from build123d import *
from build123d.topology import SkipClean

# Parameters (mm, degrees)
BOSS_EXTRUDE1_DEPTH = 25
FILLET1_R           = 2
SKETCH2_R           = 17.5
BOSS_EXTRUDE2_DEPTH = 8
SKETCH3_R           = 16.5
BOSS_EXTRUDE3_DEPTH = 12
SKETCH4_R           = 14.5
CUT_EXTRUDE1_DEPTH  = 2
SKETCH5_R           = 16.5
BOSS_EXTRUDE4_DEPTH = 1
SKETCH6_R           = 2.5
CUT_EXTRUDE2_DEPTH  = 0.75
CUT_EXTRUDE3_DEPTH  = 0.5
CUT_EXTRUDE4_DEPTH  = 0.25
SKETCH11_R          = 5
BOSS_EXTRUDE5_DEPTH = 2
BOSS_EXTRUDE6_DEPTH = 1


with BuildPart() as part:
    # Sketch1 → Boss-Extrude1 (new body)
    with BuildSketch(Plane.XY):
        with BuildLine():
            Line((-32, -20), (32, -20))
            ThreePointArc((32, -20), (34.121320344, -19.121320344), (35, -17))
            Line((35, -17), (35, 17))
            ThreePointArc((35, 17), (34.121320344, 19.121320344), (32, 20))
            Line((32, 20), (-32, 20))
            ThreePointArc((-32, 20), (-34.121320344, 19.121320344), (-35, 17))
            Line((-35, 17), (-35, -17))
            ThreePointArc((-35, -17), (-34.121320344, -19.121320344), (-32, -20))
        make_face()
    extrude(amount=BOSS_EXTRUDE1_DEPTH)

    # Fillet1
    fillet1_edges = [part.edges().sort_by_distance(p)[0] for p in [
        (0, -20, 0),
        (-34.121320344, -19.121320344, 0),
        (-35, 0, 0),
        (-34.121320344, 19.121320344, 0),
        (-34.121320344, -19.121320344, 25),
        (0, -20, 25),
        (34.121320344, -19.121320344, 25),
        (35, 0, 25),
        (34.121320344, 19.121320344, 25),
        (0, 20, 25),
        (-34.121320344, 19.121320344, 25),
        (0, 20, 0),
        (-35, 0, 25),
        (34.121320344, 19.121320344, 0),
        (35, 0, 0),
        (34.121320344, -19.121320344, 0),
    ]]
    fillet(fillet1_edges, radius=FILLET1_R)

    # Sketch2 → Boss-Extrude2 (add)
    with BuildSketch(Plane.XY.offset(25)):
        with Locations(Location((0, 0, 0), (0, 0, 180))):
            Circle(SKETCH2_R)
    extrude(amount=BOSS_EXTRUDE2_DEPTH)

    # Sketch3 → Boss-Extrude3 (add)
    with BuildSketch(Plane.XY.offset(33)):
        Circle(SKETCH3_R)
    extrude(amount=BOSS_EXTRUDE3_DEPTH)

    # Sketch4 → Cut-Extrude1 (cut)
    with BuildSketch(Plane.XY.offset(45)):
        Circle(SKETCH4_R)
    extrude(amount=-CUT_EXTRUDE1_DEPTH, mode=Mode.SUBTRACT)

    # Sketch5 → Boss-Extrude4 (add)
    with BuildSketch(Plane.XY.offset(43)):
        Circle(SKETCH5_R)
    extrude(amount=BOSS_EXTRUDE4_DEPTH)

    # Sketch6 → Cut-Extrude2 (cut)
    with BuildSketch(Plane(origin=(0, 0, 0), x_dir=(-1, 0, 0), z_dir=(0, 0, -1))):
        with Locations((-25, 13.28125)):
            Circle(SKETCH6_R)
        with Locations(Location((25, 13.28125, 0), (0, 0, 180))):
            Circle(SKETCH6_R)
        with Locations((25, -13.28125)):
            Circle(SKETCH6_R)
        with Locations(Location((-25, -13.28125, 0), (0, 0, 180))):
            Circle(SKETCH6_R)
    extrude(amount=-CUT_EXTRUDE2_DEPTH, mode=Mode.SUBTRACT)

    # Sketch7 → Cut-Extrude3 (cut)
    with SkipClean():  # the faces are left unmerged after this step: merging them gives an invalid solid
        with BuildSketch(Plane(origin=(0, 0, 0.75), x_dir=(-1, 0, 0), z_dir=(0, 0, -1))):
            with BuildLine():
                Line((-24.6, 15.749042536), (-24.6, 13.68125))
                Line((-24.6, 13.68125), (-22.532207464, 13.68125))
                ThreePointArc((-22.532207464, 13.68125), (-22.5, 13.28125), (-22.532207464, 12.88125))
                Line((-22.532207464, 12.88125), (-24.6, 12.88125))
                Line((-24.6, 12.88125), (-24.6, 10.813457464))
                ThreePointArc((-24.6, 10.813457464), (-25, 10.78125), (-25.4, 10.813457464))
                Line((-25.4, 10.813457464), (-25.4, 12.88125))
                Line((-25.4, 12.88125), (-27.467792536, 12.88125))
                ThreePointArc((-27.467792536, 12.88125), (-27.5, 13.28125), (-27.467792536, 13.68125))
                Line((-27.467792536, 13.68125), (-25.4, 13.68125))
                Line((-25.4, 13.68125), (-25.4, 15.749042536))
                ThreePointArc((-25.4, 15.749042536), (-25, 15.78125), (-24.6, 15.749042536))
            make_face()
            with BuildLine():
                Line((25.4, 13.68125), (25.4, 15.749042536))
                ThreePointArc((25.4, 15.749042536), (25, 15.78125), (24.6, 15.749042536))
                Line((24.6, 15.749042536), (24.6, 13.68125))
                Line((24.6, 13.68125), (22.532207464, 13.68125))
                ThreePointArc((22.532207464, 13.68125), (22.5, 13.28125), (22.532207464, 12.88125))
                Line((22.532207464, 12.88125), (24.6, 12.88125))
                Line((24.6, 12.88125), (24.6, 10.813457464))
                ThreePointArc((24.6, 10.813457464), (25, 10.78125), (25.4, 10.813457464))
                Line((25.4, 10.813457464), (25.4, 12.88125))
                Line((25.4, 12.88125), (27.467792536, 12.88125))
                ThreePointArc((27.467792536, 12.88125), (27.5, 13.28125), (27.467792536, 13.68125))
                Line((27.467792536, 13.68125), (25.4, 13.68125))
            make_face()
            with BuildLine():
                Line((24.6, -15.749042536), (24.6, -13.68125))
                Line((24.6, -13.68125), (22.532207464, -13.68125))
                ThreePointArc((22.532207464, -13.68125), (22.5, -13.28125), (22.532207464, -12.88125))
                Line((22.532207464, -12.88125), (24.6, -12.88125))
                Line((24.6, -12.88125), (24.6, -10.813457464))
                ThreePointArc((24.6, -10.813457464), (25, -10.78125), (25.4, -10.813457464))
                Line((25.4, -10.813457464), (25.4, -12.88125))
                Line((25.4, -12.88125), (27.467792536, -12.88125))
                ThreePointArc((27.467792536, -12.88125), (27.5, -13.28125), (27.467792536, -13.68125))
                Line((27.467792536, -13.68125), (25.4, -13.68125))
                Line((25.4, -13.68125), (25.4, -15.749042536))
                ThreePointArc((25.4, -15.749042536), (25, -15.78125), (24.6, -15.749042536))
            make_face()
            with BuildLine():
                Line((-25.4, -13.68125), (-25.4, -15.749042536))
                ThreePointArc((-25.4, -15.749042536), (-25, -15.78125), (-24.6, -15.749042536))
                Line((-24.6, -15.749042536), (-24.6, -13.68125))
                Line((-24.6, -13.68125), (-22.532207464, -13.68125))
                ThreePointArc((-22.532207464, -13.68125), (-22.5, -13.28125), (-22.532207464, -12.88125))
                Line((-22.532207464, -12.88125), (-24.6, -12.88125))
                Line((-24.6, -12.88125), (-24.6, -10.813457464))
                ThreePointArc((-24.6, -10.813457464), (-25, -10.78125), (-25.4, -10.813457464))
                Line((-25.4, -10.813457464), (-25.4, -12.88125))
                Line((-25.4, -12.88125), (-27.467792536, -12.88125))
                ThreePointArc((-27.467792536, -12.88125), (-27.5, -13.28125), (-27.467792536, -13.68125))
                Line((-27.467792536, -13.68125), (-25.4, -13.68125))
            make_face()
        extrude(amount=-CUT_EXTRUDE3_DEPTH, mode=Mode.SUBTRACT)

    # Sketch8 → Cut-Extrude4 (cut)
    with SkipClean():  # the faces are left unmerged after this step: merging them gives an invalid solid
        with BuildSketch(Plane(origin=(0, 20, 0), x_dir=(1, 0, 0), z_dir=(0, 1, 0))):
            with BuildLine():
                Line((26, -18), (13, -18))
                ThreePointArc((13, -18), (12.292893219, -17.707106781), (12, -17))
                Line((12, -17), (12, -11))
                ThreePointArc((12, -11), (12.292893219, -10.292893219), (13, -10))
                Line((13, -10), (26, -10))
                ThreePointArc((26, -10), (26.707106781, -10.292893219), (27, -11))
                Line((27, -11), (27, -17))
                ThreePointArc((27, -17), (26.707106781, -17.707106781), (26, -18))
            make_face()
        extrude(amount=-CUT_EXTRUDE4_DEPTH, mode=Mode.SUBTRACT)

    # Sketch11 → Boss-Extrude5 (add)
    with SkipClean():  # the faces are left unmerged after this step: merging them gives an invalid solid
        with BuildSketch(Plane.ZY.offset(35)):
            with Locations(Location((12.5, 0, 0), (0, 0, 180))):
                Circle(SKETCH11_R)
        boss_extrude5 = extrude(amount=BOSS_EXTRUDE5_DEPTH)

    # Mirror1: Boss-Extrude5 across plane
    with SkipClean():  # the faces are left unmerged after this step: merging them gives an invalid solid
        add(boss_extrude5.mirror(Plane(origin=(0, 0, 0), x_dir=(0, 0, 1), z_dir=(1, 0, 0))))

    # Sketch12 → Boss-Extrude6 (add)
    with SkipClean():  # the faces are left unmerged after this step: merging them gives an invalid solid
        with BuildSketch(Plane.XY.offset(25)):
            with BuildLine():
                Line((25.5, 14), (29.5, 14))
                ThreePointArc((29.5, 14), (29.853553391, 13.853553391), (30, 13.5))
                Line((30, 13.5), (30, 12))
                ThreePointArc((30, 12), (29.853553391, 11.646446609), (29.5, 11.5))
                Line((29.5, 11.5), (25.5, 11.5))
                ThreePointArc((25.5, 11.5), (25.146446609, 11.646446609), (25, 12))
                Line((25, 12), (25, 13.5))
                ThreePointArc((25, 13.5), (25.146446609, 13.853553391), (25.5, 14))
            make_face()
        extrude(amount=BOSS_EXTRUDE6_DEPTH)


solid = part.part
Work out the finished part from the listing and answer in its coordinate system (mm). A direction names the side the tool comes from. Give positions to 0.01 mm unless a question says otherwise; leave off trailing zeros. Loops run counter-clockwise (first coordinate to the right, second up) from the corner with the lowest first, then second, coordinate; pieces in that order, holes last. Notation, with made-up numbers: (19, 43.5) - (59, 43.5) arc R22 cw to (59, 64.5) - close; hole circle Ø3 at (-28, 81). An arc over 180 degrees is marked (long way). Answer in a Markdown table with one row per item.
(1) Section A-A (z = 12.5) is taken. Give the vertices of the cut face in (x, y).
Results list:
| item | result |
|---|---|
| outline | (-37, -5) - (-35, -5) - (-35, -17) arc R3 ccw to (-32, -20) - (32, -20) arc R3 ccw to (35, -17) - (35, -5) - (37, -5) - (37, 5) - (35, 5) - (35, 17) arc R3 ccw to (32, 20) - (27, 20) - (27, 19.75) - (12, 19.75) - (12, 20) - (-32, 20) arc R3 ccw to (-35, 17) - (-35, 5) - (-37, 5) - close |
(2) A tool of negligible diameter and unlimited length cuts with its end or side. For faces 5 (the face through (5, -16, 33)), 6 (the face through (-26, 12, 0.75)), 7 (the face through (35.99, -1.5, 7.73)), from which of +Z, -Z, +X, -X, +Y, -Y can it reach the whole face along a straight path? Write none if from no direction.
Results list:
| item | result |
|---|---|
| face 5 | +Z |
| face 6 | -Z |
| face 7 | +X |
(3) For a pull along X with two mould halves and no side action, classify faces 1 (the face through (-34.43, -0.24, 0.6)), 2 (the face through (-26, -14, 0.75)), 3 (the face through (0, 20, 12)), 4 (the face through (26, -12, 0.75)) as pulls with the +X half, pulls with the -X half, needs draft (parallel to the pull), parting line crosses it, or undercut.
Results list:
| item | result |
|---|---|
| face 1 | pulls with the -X half |
| face 2 | undercut |
| face 3 | needs draft |
| face 4 | undercut |
(4) Section C-C (x = 21) is taken. Give the vertices of the cut face in (y, z).
Results list:
| item | result |
|---|---|
| outline | (-20, 2) arc R2 ccw to (-18, 0) - (18, 0) arc R2 ccw to (20, 2) - (20, 10) - (19.75, 10) - (19.75, 18) - (20, 18) - (20, 23) arc R2 ccw to (18, 25) - (-18, 25) arc R2 ccw to (-20, 23) - close |
(5) Section D-D (y = -9) is taken. Give the vertices of the cut face in (x, z).
Results list:
| item | result |
|---|---|
| outline | (-35, 2) arc R2 ccw to (-33, 0) - (33, 0) arc R2 ccw to (35, 2) - (35, 23) arc R2 ccw to (33, 25) - (15.01, 25) - (15.01, 33) - (13.83, 33) - (13.83, 45) - (11.37, 45) - (11.37, 44) - (-11.37, 44) - (-11.37, 45) - (-13.83, 45) - (-13.83, 33) - (-15.01, 33) - (-15.01, 25) - (-33, 25) arc R2 ccw to (-35, 23) - close |
(6) Consider L1, parallel to Y at x = 25, z = 0.2; L2, parallel to Y at x = 0, z = 44.5; L3, parallel to X at y = 15, z = 23. Determine where each line is inside the solid, lowest interval first. Write a range as [from, to].
Results list:
| item | result |
|---|---|
| L1 | y = [-18.87, -15.78], [-10.78, 10.78], [15.78, 18.87] |
| L2 | y = [-16.5, -14.5], [14.5, 16.5] |
| L3 | x = [-35, 35] |
(7) Section B-B (y = 0) is taken. Give the vertices of the cut face in (x, z).
Results list:
| item | result |
|---|---|
| outline | (-37, 7.5) - (-35, 7.5) - (-35, 2) arc R2 ccw to (-33, 0) - (33, 0) arc R2 ccw to (35, 2) - (35, 7.5) - (37, 7.5) - (37, 17.5) - (35, 17.5) - (35, 23) arc R2 ccw to (33, 25) - (17.5, 25) - (17.5, 33) - (16.5, 33) - (16.5, 45) - (14.5, 45) - (14.5, 44) - (-14.5, 44) - (-14.5, 45) - (-16.5, 45) - (-16.5, 33) - (-17.5, 33) - (-17.5, 25) - (-33, 25) arc R2 ccw to (-35, 23) - (-35, 17.5) - (-37, 17.5) - close |
(8) Flat-ended cylindrical pins translate along their axes: pin 1 Ø4 at (x, y) = (5, -5) entering from +Z; pin 2 Ø8 at (y, z) = (-6, 40.5) entering from +X; pin 3 Ø1.5 at (x, y) = (-25, 14.5) entering from -Z. Find the tip coordinate at first contact, or state that the pin passes through.
Results list:
| item | result |
|---|---|
| pin 1 | stops at z = 44 |
| pin 2 | stops at x = 16.38 |
| pin 3 | stops at z = 0.75 |
